Source: CAD feature listing. Evaluate the final solid. Frame: model axes, mm. Face numbers are marked on the shaded views. A direction names the side the tool comes from. Coordinates: 2 decimals unless noted, no trailing zeros. Write each loop counter-clockwise with the first axis right and the second up, starting at its lowest first coordinate (ties: lowest second). Pieces come first, ordered by that corner, then holes. Notation, with made-up numbers: M -3.75,19.5 L 32.25,19.5 A36 ccw 32.25,54.5 Z; hole C -35.75,-35 d1. An arc over 180 degrees is marked long. One line per item, written item: value. Start each with the question number.
Item 1: Mould query, pull axis X, two halves, no side actions, for the marked faces 1, 2, 3 and 4. Classes: released by +X, released by -X, zero draft, split by the parting line, or undercut.
Item 2: Cut plane D-D, the plane y = 2.75. Output: boundary loops of the cut face in (x, z), then the cut area to 3 significant figures.
Item 3: Cut plane C-C, the plane x = 8. Output: boundary loops of the cut face in (y, z), then the cut area to 3 significant figures.
Item 4: Ray query, L1, parallel to X at y = 13.5, z = 31.5; L2, parallel to Z at x = -13.25, y = 9.5; L3, parallel to Y at x = -4, z = 24.5. Return the intervals inside material, ascending. Write a range as from..to.
Item 5: Cut plane B-B, the plane y = 15.25. Output: boundary loops of the cut face in (x, z), then the cut area to 3 significant figures.
Item 6: Pin query (flat end, axial travel): P1, Ø5.5, axis at y = 9, z = 45.5, coming from the +X side; P2, Ø3, axis at x = 16, y = 7.5, coming from the +Z side; P3, Ø10.5, axis at x = 8, z = 16.5, coming from the +Y side; P4, Ø3, axis at y = 9.5, z = 48.92, coming from the -X side. Return the tip coordinate at first contact, or that it passes through.
Item 7: Cut plane A-A, the plane z = 6.5. Output: boundary loops of the cut face in (x, y), then the cut area to 3 significant figures.
Item 8: Set-up query: the marked faces 5, 6, 7, 8 and 9. Return all of +Z, -Z, +X, -X, +Y, -Y with unobstructed straight access to the full face (end or side cutting, diameter ignored); none if empty.
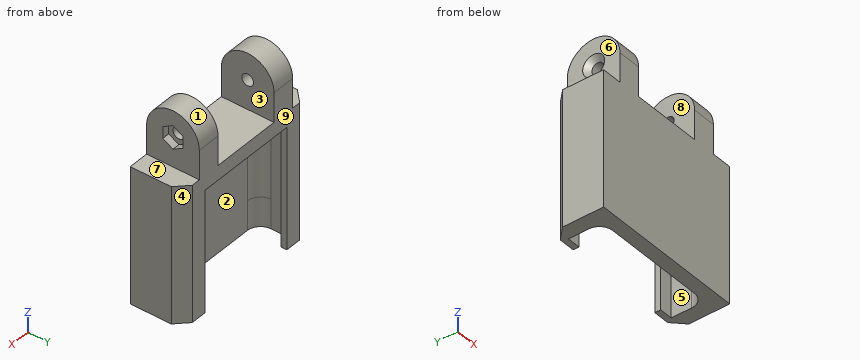
```python
from build123d import *

# Parameters (mm, degrees)
SKETCH1_W                     = 56
SKETCH1_H                     = 45
BOSS_EXTRUDE1_DEPTH           = 5
BOSS_EXTRUDE2_DEPTH           = 5
SKETCH3_W                     = 56
SKETCH3_H                     = 8.40027106
CUT_EXTRUDE1_DEPTH            = 0.5
BOSS_EXTRUDE3_DEPTH           = 3.5
SKETCH5_W                     = 5
SKETCH5_H                     = 3.247037966
CUT_EXTRUDE2_DEPTH            = 3.5
BOSS_EXTRUDE4_DEPTH           = 16.416410101
BOSS_EXTRUDE5_DEPTH           = 54
CHAMFER1_SIZE                 = 4
CSK_FOR_M4_SFHCS1_D           = 4
CSK_FOR_M4_SFHCS1_DEPTH       = 5
CSK_FOR_M4_SFHCS1_CSINK_D     = 7.6
CSK_FOR_M4_SFHCS1_CSINK_ANGLE = 90
CUT_EXTRUDE3_DEPTH            = 80.660134165
CUT_EXTRUDE3_DEPTH_BACK       = 80.660134165
SKETCH11_W                    = 8
SKETCH11_H                    = 16.218738619
FILLET1_R                     = 4.5
CUT_EXTRUDE4_START            = 18
CUT_EXTRUDE4_DEPTH            = 18
BOSS_EXTRUDE6_DEPTH           = 18
BOSS_EXTRUDE7_START           = -90
BOSS_EXTRUDE7_DEPTH           = 18
SKETCH16_W                    = 118.653956423
SKETCH16_H                    = 92.574487852
CUT_EXTRUDE5_DEPTH            = 39
SKETCH17_W                    = 131.858911514
SKETCH17_H                    = 83.404733186
CUT_EXTRUDE6_DEPTH            = 86
SKETCH18_W                    = 99.193977615
SKETCH18_H                    = 87.816890576
CUT_EXTRUDE7_DEPTH            = 109
SKETCH19_W                    = 81.935577426
SKETCH19_H                    = 38.938723706
CUT_EXTRUDE8_DEPTH            = 24.977359313
BOSS_EXTRUDE8_START           = 10
BOSS_EXTRUDE8_DEPTH           = 10
BOSS_EXTRUDE9_DEPTH           = 5
SKETCH22_W                    = 8
SKETCH22_H                    = 18
BOSS_EXTRUDE10_DEPTH          = 10
BOSS_EXTRUDE11_START          = -8
BOSS_EXTRUDE11_DEPTH          = 8
BOSS_EXTRUDE12_START          = -40
BOSS_EXTRUDE12_DEPTH          = 8
CSK_FOR_M4_SFHCS2_D           = 4
CSK_FOR_M4_SFHCS2_DEPTH       = 40
CSK_FOR_M4_SFHCS2_CSINK_D     = 7.5
CSK_FOR_M4_SFHCS2_CSINK_ANGLE = 90
CSK_FOR_M4_SFHCS2_TIP         = 1.201721238
CUT_EXTRUDE9_DEPTH            = 2.5


with BuildPart() as part:
    # Sketch1 → Boss-Extrude1 (new body)
    with BuildSketch(Plane(origin=(0, 0, 0), x_dir=(1, 0, 0), z_dir=(0, 1, 0))):
        Rectangle(SKETCH1_W, SKETCH1_H)
    extrude(amount=BOSS_EXTRUDE1_DEPTH)

    # Sketch2 → Boss-Extrude2 (add)
    with BuildSketch(Plane.XZ):
        Polygon((-45, -6.940200144), (-24, 6.697359313), (24, 6.697359313), (45, -6.940200144), (45, 3.059799856), (28, 14.09972894), (-28, 14.09972894), (-45, 3.059799856), align=None)
    extrude(amount=BOSS_EXTRUDE2_DEPTH)

    # Sketch3 → Cut-Extrude1 (cut)
    with BuildSketch(Plane.XZ):
        with Locations((0, 18.29986447)):
            Rectangle(SKETCH3_W, SKETCH3_H)
    extrude(amount=-CUT_EXTRUDE1_DEPTH, mode=Mode.SUBTRACT)

    # Sketch4 → Boss-Extrude3 (add)
    with BuildSketch(Plane(origin=(0, 0, 0), x_dir=(1, 0, 0), z_dir=(0, 1, 0))):
        Polygon((28, -40.539929084), (28, 22.5), (45, 22.5), (45, -29.5), align=None)
        Polygon((-28, -4.09972894), (-28, 22.5), (-45, 22.5), (-45, 6.940200144), align=None)
        Polygon((-28, -40.539929084), (-28, -14.09972894), (-45, -3.059799856), (-45, -29.5), align=None)
        Polygon((-45, -3.059799856), (-28, -14.09972894), (-28, -4.09972894), (-45, 6.940200144), align=None)
    extrude(amount=BOSS_EXTRUDE3_DEPTH)

    # Sketch5 → Cut-Extrude2 (cut)
    with BuildSketch(Plane(origin=(0, 3.5, 0), x_dir=(1, 0, 0), z_dir=(0, 1, 0))):
        with Locations((-28, -40.539929084)):
            Rectangle(SKETCH5_W, SKETCH5_H)
        with Locations((28, -40.539929084)):
            Rectangle(SKETCH5_W, SKETCH5_H)
    extrude(amount=-CUT_EXTRUDE2_DEPTH, mode=Mode.SUBTRACT)

    # Sketch6 → Boss-Extrude4 (add)
    with BuildSketch(Plane.XY.offset(22.5)):
        Polygon((-28, 0.5), (28, 0.5), (28, 3.5), (28, 5), (-28, 5), (-28, 3.5), align=None)
    extrude(amount=BOSS_EXTRUDE4_DEPTH)

    # Sketch8 → Boss-Extrude5 (add)
    with BuildSketch(Plane.XY.offset(38.916410101)):
        Polygon((-22, 5), (-22, 16.5), (-17.5, 16.5), (-17.5, 18.5), (-27, 18.5), (-27, 16.5), (-27, 5), align=None)
        Polygon((27, 5), (27, 16.5), (27, 18.5), (17.5, 18.5), (17.5, 16.5), (22, 16.5), (22, 5), align=None)
    extrude(amount=-BOSS_EXTRUDE5_DEPTH)

    # Chamfer1
    chamfer1_edges = [part.edges().sort_by_distance(p)[0] for p in [
        (-27, 18.5, 11.916410101),
        (27, 18.5, 11.916410101),
    ]]
    chamfer(chamfer1_edges, length=CHAMFER1_SIZE)

    # CSK for M4 SFHCS1
    with Locations(Plane(origin=(0, 5, 0), x_dir=(1, 0, 0), z_dir=(0, 1, 0))):
        with Locations((-17, 1.522640687), (17, 1.522640687)):
            CounterSinkHole(CSK_FOR_M4_SFHCS1_D / 2, CSK_FOR_M4_SFHCS1_CSINK_D / 2, depth=CSK_FOR_M4_SFHCS1_DEPTH, counter_sink_angle=CSK_FOR_M4_SFHCS1_CSINK_ANGLE)

    # Sketch11 → Cut-Extrude3 (cut, two sides: drawn at the far end of the back side and taken through both)
    with BuildSketch(Plane.ZY.offset(-22).offset(-CUT_EXTRUDE3_DEPTH_BACK)):
        with Locations((-1.522640687, 13.109369309)):
            Rectangle(SKETCH11_W, SKETCH11_H)
    extrude(amount=CUT_EXTRUDE3_DEPTH + CUT_EXTRUDE3_DEPTH_BACK, mode=Mode.SUBTRACT)

    # Fillet1
    fillet1_edges = [part.edges().sort_by_distance(p)[0] for p in [
        (-22, 5, -10.303115293),
        (22, 5, -10.303115293),
        (-22, 5, 20.696884707),
        (22, 5, 20.696884707),
    ]]
    fillet(fillet1_edges, radius=FILLET1_R)

    # Sketch14 → Cut-Extrude4 (cut)
    with BuildSketch(Plane(origin=(0, 0, 2.477359313), x_dir=(-1, 0, 0), z_dir=(0, 0, -1)).offset(CUT_EXTRUDE4_START)):
        with BuildLine():
            Line((-27, 5), (-17.5, 5))
            ThreePointArc((-17.5, 5), (-20.681980515, 6.318019485), (-22, 9.5))
            Line((-22, 9.5), (-22, 16.5))
            Line((-22, 16.5), (-17.5, 16.5))
            Line((-17.5, 16.5), (-17.5, 18.5))
            Line((-17.5, 18.5), (-23, 18.5))
            Line((-23, 18.5), (-27, 14.5))
            Line((-27, 14.5), (-27, 5))
        make_face()
        with BuildLine():
            Line((22, 16.5), (22, 9.5))
            ThreePointArc((22, 9.5), (20.681980515, 6.318019485), (17.5, 5))
            Line((17.5, 5), (27, 5))
            Line((27, 5), (27, 14.5))
            Line((27, 14.5), (23, 18.5))
            Line((23, 18.5), (17.5, 18.5))
            Line((17.5, 18.5), (17.5, 16.5))
            Line((17.5, 16.5), (22, 16.5))
        make_face()
    extrude(amount=-CUT_EXTRUDE4_DEPTH, mode=Mode.SUBTRACT)

    # Sketch15 → Boss-Extrude6 (add)
    with BuildSketch(Plane.ZY.offset(45)):
        Polygon((29.5, 3.5), (49.5, 3.5), (60.311407923, -47.363675238), (55.199704948, -47.363675238), (45.132244992, 0), (29.5, 0), align=None)
    extrude(amount=-BOSS_EXTRUDE6_DEPTH)

    # Sketch15<3> → Boss-Extrude7 (add)
    with BuildSketch(Plane.ZY.offset(45).offset(BOSS_EXTRUDE7_START)):
        Polygon((29.5, 3.5), (49.5, 3.5), (60.311407923, -47.363675238), (55.199704948, -47.363675238), (45.132244992, 0), (29.5, 0), align=None)
    extrude(amount=BOSS_EXTRUDE7_DEPTH)

    # Sketch16 → Cut-Extrude5 (cut)
    with BuildSketch(Plane.ZY.offset(27)):
        with Locations((22.108445716, -11.305351621)):
            Rectangle(SKETCH16_W, SKETCH16_H)
    extrude(amount=CUT_EXTRUDE5_DEPTH, mode=Mode.SUBTRACT)

    # Sketch17 → Cut-Extrude6 (cut)
    with BuildSketch(Plane(origin=(27, 0, 0), x_dir=(0, 0, -1), z_dir=(1, 0, 0))):
        with Locations((-19.541168595, -14.670136857)):
            Rectangle(SKETCH17_W, SKETCH17_H)
    extrude(amount=CUT_EXTRUDE6_DEPTH, mode=Mode.SUBTRACT)

    # Sketch18 → Cut-Extrude7 (cut)
    with BuildSketch(Plane.XZ.offset(-0.5)):
        with Locations((2.429482128, 7.437881449)):
            Rectangle(SKETCH18_W, SKETCH18_H)
    extrude(amount=CUT_EXTRUDE7_DEPTH, mode=Mode.SUBTRACT)

    # Sketch19 → Cut-Extrude8 (cut)
    with BuildSketch(Plane(origin=(0, 0, -22.5), x_dir=(-1, 0, 0), z_dir=(0, 0, -1))):
        with Locations((6.570305737, 10.128043931)):
            Rectangle(SKETCH19_W, SKETCH19_H)
    extrude(amount=-CUT_EXTRUDE8_DEPTH, mode=Mode.SUBTRACT)

    # Sketch20 → Boss-Extrude8 (add)
    with BuildSketch(Plane(origin=(0, 0, 2.477359313), x_dir=(-1, 0, 0), z_dir=(0, 0, -1)).offset(BOSS_EXTRUDE8_START)):
        with BuildLine():
            Line((-27, 14.5), (-27, 0.5))
            Line((-27, 0.5), (27, 0.5))
            Line((27, 0.5), (27, 14.5))
            Line((27, 14.5), (23, 18.5))
            Line((23, 18.5), (17.5, 18.5))
            Line((17.5, 18.5), (17.5, 16.5))
            Line((17.5, 16.5), (22, 16.5))
            Line((22, 16.5), (22, 9.5))
            ThreePointArc((22, 9.5), (20.681980515, 6.318019485), (17.5, 5))
            Line((17.5, 5), (-17.5, 5))
            ThreePointArc((-17.5, 5), (-20.681980515, 6.318019485), (-22, 9.5))
            Line((-22, 9.5), (-22, 16.5))
            Line((-22, 16.5), (-17.5, 16.5))
            Line((-17.5, 16.5), (-17.5, 18.5))
            Line((-17.5, 18.5), (-23, 18.5))
            Line((-23, 18.5), (-27, 14.5))
        make_face()
    extrude(amount=-BOSS_EXTRUDE8_DEPTH)

    # Sketch21 → Boss-Extrude9 (add)
    with BuildSketch(Plane.XY.offset(38.916410101)):
        Polygon((17.5, 18.5), (-17.5, 18.5), (-23, 18.5), (-27, 14.5), (-27, 0.5), (27, 0.5), (27, 14.5), (23, 18.5), align=None)
    extrude(amount=-BOSS_EXTRUDE9_DEPTH)

    # Sketch22 → Boss-Extrude10 (add)
    with BuildSketch(Plane.XY.offset(38.916410101)):
        with Locations((-16, 9.5)):
            Rectangle(SKETCH22_W, SKETCH22_H)
        with Locations((16, 9.5)):
            Rectangle(SKETCH22_W, SKETCH22_H)
    extrude(amount=BOSS_EXTRUDE10_DEPTH)

    # Sketch23 → Boss-Extrude11 (add)
    with BuildSketch(Plane(origin=(20, 0, 0), x_dir=(0, 0, -1), z_dir=(1, 0, 0)).offset(BOSS_EXTRUDE11_START)):
        with BuildLine():
            Line((-48.916410101, 18.5), (-48.916410101, 0.5))
            ThreePointArc((-48.916410101, 0.5), (-57.916410101, 9.5), (-48.916410101, 18.5))
        make_face()
    extrude(amount=BOSS_EXTRUDE11_DEPTH)

    # Sketch23<2> → Boss-Extrude12 (add)
    with BuildSketch(Plane(origin=(20, 0, 0), x_dir=(0, 0, -1), z_dir=(1, 0, 0)).offset(BOSS_EXTRUDE12_START)):
        with BuildLine():
            Line((-48.916410101, 18.5), (-48.916410101, 0.5))
            ThreePointArc((-48.916410101, 0.5), (-57.916410101, 9.5), (-48.916410101, 18.5))
        make_face()
    extrude(amount=BOSS_EXTRUDE12_DEPTH)

    # CSK for M4 SFHCS2
    with Locations(Plane.ZY.offset(20)):
        with Locations((48.916410101, 9.5)):
            CounterSinkHole(CSK_FOR_M4_SFHCS2_D / 2, CSK_FOR_M4_SFHCS2_CSINK_D / 2, depth=CSK_FOR_M4_SFHCS2_DEPTH, counter_sink_angle=CSK_FOR_M4_SFHCS2_CSINK_ANGLE)
            with Locations((0, 0, -(CSK_FOR_M4_SFHCS2_DEPTH + CSK_FOR_M4_SFHCS2_TIP / 2))):  # 118° drill point
                Cone(0, CSK_FOR_M4_SFHCS2_D / 2, CSK_FOR_M4_SFHCS2_TIP, mode=Mode.SUBTRACT)

    # Sketch27 → Cut-Extrude9 (cut)
    with BuildSketch(Plane(origin=(20, 0, 0), x_dir=(0, 0, -1), z_dir=(1, 0, 0))):
        Polygon((-44.932693244, 9.5), (-46.924551673, 12.95), (-50.90826853, 12.95), (-52.900126959, 9.5), (-50.90826853, 6.05), (-46.924551673, 6.05), align=None)
    extrude(amount=-CUT_EXTRUDE9_DEPTH, mode=Mode.SUBTRACT)


solid = part.part
```
From the geometry:
1. face 1: zero draft
1. face 2: undercut
1. face 3: undercut
1. face 4: released by +X
2. outline: M -27,-7.52 L 27,-7.52 L 27,38.92 L 20,38.92 L 20,54.87 L 12,54.87 L 12,38.92 L -12,38.92 L -12,54.87 L -20,54.87 L -20,38.92 L -27,38.92 Z
2. area: 2,760 mm²
3. outline: M 0.5,-7.52 L 5,-7.52 L 5,33.92 L 18.5,33.92 L 18.5,38.92 L 0.5,38.92 Z
3. area: 276 mm²
4. L1: x = -27..-22, 22..27
4. L2: z = 33.92..46.92, 50.92..57.92
4. L3: y = 0.5..5
5. outline: M -26.25,-7.52 L -22,-7.52 L -22,33.92 L 22,33.92 L 22,-7.52 L 26.25,-7.52 L 26.25,38.92 L 20,38.92 L 20,55.84 L 12,55.84 L 12,38.92 L -12,38.92 L -12,55.84 L -20,55.84 L -20,38.92 L -26.25,38.92 Z
5. area: 886 mm²
6. P1: stops at x = 20
6. P2: stops at z = 57.9
6. P3: stops at y = 5
6. P4: passes through
7. outline: M -27,0.5 L 27,0.5 L 27,14.5 L 23,18.5 L 17.5,18.5 L 17.5,16.5 L 22,16.5 L 22,9.5 A4.5 cw 17.5,5 L -17.5,5 A4.5 cw -22,9.5 L -22,16.5 L -17.5,16.5 L -17.5,18.5 L -23,18.5 L -27,14.5 Z
7. area: 389 mm²
8. face 5: -Z
8. face 6: +Z, -X, +Y, -Y
8. face 7: +Z, +X, +Y, -Y
8. face 8: +Z, +Y, -Y
8. face 9: +Z, -Z, +X, -X, +Y
